Verification items for the finished model (mm, model axes). Face numbers are marked on the shaded views. Round coordinates to 2 decimals unless told otherwise and drop trailing zeros. Order: outer loops, then holes, each group sorted by start corner. A loop starts at its lowest first (then second) coordinate and runs counter-clockwise, first axis right, second up. Notation, with made-up numbers: M -9,-31 L 46,-31 A10 ccw 46,-17 Z; hole C 63,61.25 d5. An arc over 180 degrees is marked long. Return JSON: item names as keys, results as strings. Group by question number.
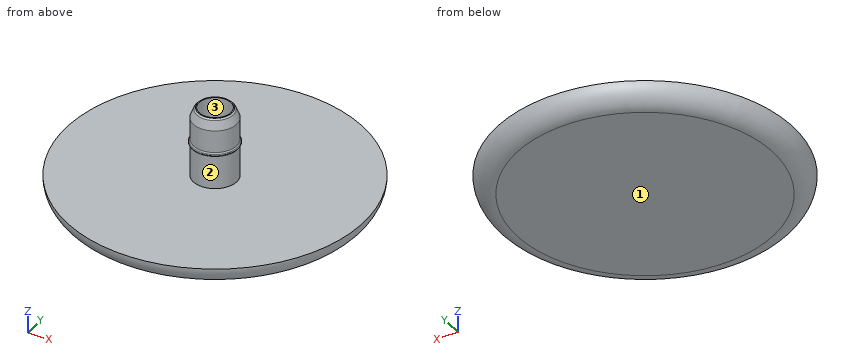
from build123d import *

# Parameters (mm, degrees)
F0_R     = 2.2
F1_DEPTH = 7
F2_T     = -0.6
F0_R_2   = 15
F3_DEPTH = 2
F4_R     = 1.99999
F7_SIZE  = 0.5
F8_SIZE  = 0.5
F9_R     = 0.2


# Not quite as in the source:
# - a fillet or chamfer is up to 0.001 mm smaller than in the source, because OpenCascade refuses the exact size


with BuildPart() as f1:
    # F0 (on Top) → F1 (new body)
    with BuildSketch(Plane.XY):
        Circle(F0_R)
    extrude(amount=F1_DEPTH)

    # F2
    f2_openings = [f1.faces().sort_by_distance(p)[0] for p in [
        (0, 0, 7),
    ]]
    offset(amount=F2_T, openings=f2_openings)

    # F0 (on Top) → F3 (join)
    with BuildSketch(Plane.XY):
        Circle(F0_R_2)
        Circle(F0_R, mode=Mode.SUBTRACT)
        Circle(F0_R)
    extrude(amount=-F3_DEPTH)

    # F4 (radius 2 in the source; OpenCascade refuses exactly that, so slightly less here)
    f4_edges = [f1.edges().sort_by_distance(p)[0] for p in [
        (-15, 0, -2),
    ]]
    fillet(f4_edges, radius=F4_R)

    # F5 (on Front) → F6 (revolve)
    with BuildSketch(Plane.XZ):
        with BuildLine():
            ThreePointArc((2.075, 3.5), (2.1116116524, 3.4116116524), (2.2, 3.375))
            Line((2.2, 3.375), (2.2, 3.5))
            Line((2.2, 3.5), (2.075, 3.5))
        make_face()
        with BuildLine():
            Line((2.2, 3.5), (2.2, 3.375))
            ThreePointArc((2.2, 3.375), (2.2883883476, 3.4116116524), (2.325, 3.5))
            ThreePointArc((2.325, 3.5), (2.2, 3.625), (2.075, 3.5))
            Line((2.075, 3.5), (2.2, 3.5))
        make_face()
    revolve(axis=Axis((0, 0, 1.75), (0, 0, 1)))

    # F7
    f7_edges = [f1.edges().sort_by_distance(p)[0] for p in [
        (-2.2, 0, 7),
    ]]
    chamfer(f7_edges, length=F7_SIZE)

    # F8
    f8_edges = [f1.edges().sort_by_distance(p)[0] for p in [
        (-2.2, 0, 6.5),
    ]]
    chamfer(f8_edges, length=F8_SIZE)

    # F9
    f9_edges = [f1.edges().sort_by_distance(p)[0] for p in [
        (-2.2, 0, 3.625),
    ]]
    fillet(f9_edges, radius=F9_R)


solid = f1.part
1. Draft check along Z on the marked faces 1, 2 and 3. Enter one of: +Z half, -Z half, draft (parallel to the pull), parting line (faces both ways), or undercut.
2. Go/stop test with flat-tipped pins: pin 1 (12 mm diameter, centred on x = -11, y = 9, fed in from +Z); pin 2 (1.6 mm diameter, centred on x = -0.5, y = 0.5, fed in from +Z). Record where each tip stops, or that it passes through.
3. Thickness scan on line 1 along X through (y, z) = (0, 4.75); line 2 along Z through (x, y) = (6.25, 9.75). Record the ranges inside material, lowest first. Write a range as from..to.
4. Cross-section at A-A (z = 2.25). Enter the section's corners in (x, y), plus the area to 3 significant figures.
Computed:
{
 "1": {"face 1": "-Z half", "face 2": "undercut", "face 3": "draft"},
 "2": {"pin 1": "stops at z = 0", "pin 2": "stops at z = 0.6"},
 "3": {"line 1": "x = -2.2..-1.6, 1.6..2.2", "line 2": "z = -2..0"},
 "4": {"outline": "C 0,0 d4.4; hole C 0,0 d3.2", "area": "7.16 mm²"}
}
